Source: CAD feature listing. Evaluate the final solid. Frame: model axes, mm. A direction names the side the tool comes from. Round coordinates to 2 decimals unless told otherwise and drop trailing zeros. Order: outer loops, then holes, each group sorted by start corner. A loop starts at its lowest first (then second) coordinate and runs counter-clockwise, first axis right, second up. Notation, with made-up numbers: (-21.75, 57) -> (-17.75, 57) arc R33 cw to (-17.75, 94) -> close; hole circle Ø5 at (4.25, 23.25). An arc over 180 degrees is marked (long way). Write item = value, one per line. Start each with the question number.
(1) Contact query for flat-ended pins moving along their axis: pin 1 Ø1 at (x, z) = (9, 0) entering from +Y; pin 2 Ø0.5 at (x, z) = (15, 0) entering from -Y; pin 3 Ø1.5 at (y, z) = (6, 0) entering from +X. Output: stop coordinate, or through.
(2) Reachability of faces 1 (the face through (10.445, -2.742, -0.479)), 2 (the face through (1.42, -3.03, -0.48)), 3 (the face through (-2, 5, 0)) from +Z, -Z, +X, -X, +Y, -Y: full face, straight path, thin tool, end or side. Return the list, or none.
(3) Cut plane A-A on x = 6.5. Return the cut outline in (y, z).
(4) Cut plane B-B on z = 0.55. Return the cut outline in (x, y).
(5) Cut plane C-C on y = 3. Return the cut outline in (x, z), then the cut area to 3 significant figures.
(6) Ray query, line 1 (Y direction, x = 2.25, z = -1.05); line 2 (Y direction, x = 6.5, z = -1.1); line 3 (Y direction, x = 10, z = 0.15). Return the intervals inside material, ascending.
(7) Draft query along Y for faces 4 (the face through (2.545, 12.762, -0.479)), 5 (the face through (15, 5, 0)), 6 (the face through (13, 8, -2)), 7 (the face through (13, 3, -1)). Return one class per face: released by +Y, released by -Y, zero draft, split by the parting line, or undercut.
(8) Cut plane D-D on y = 12.5. Return the cut outline in (x, z), then the cut area to 3 significant figures.
from build123d import *

# Parameters (mm, degrees)
SKETCH009_R     = 9.5
PAD006_DEPTH    = 3
SKETCH010_R     = 6.8
POCKET003_DEPTH = 5
SKETCH013_W     = 1.6
SKETCH013_H     = 3
GROOVE_ANGLE    = -63
SKETCH014_W     = 1.6
SKETCH014_H     = 3
GROOVE001_ANGLE = -63


with BuildPart() as part:
    # Sketch009 → Pad006 (new body)
    with BuildSketch(Plane.XY.offset(1)):
        with Locations((6.5, 5)):
            Circle(SKETCH009_R)
    extrude(amount=-PAD006_DEPTH)

    # Sketch010 (on Face3 of Pad006) → Pocket003 (cut)
    with BuildSketch(Plane(origin=(0, 0, -2), x_dir=(1, 0, 0), z_dir=(0, 0, -1))):
        with Locations((6.5, -5)):
            Circle(SKETCH010_R)
    extrude(amount=-POCKET003_DEPTH, mode=Mode.SUBTRACT)

    # Sketch013 → Groove (revolve, cut)
    with BuildSketch(Plane(origin=(6.5, 5, 0), x_dir=(1, 0, 0), z_dir=(0, -1, 0))):
        with Locations((8.7, -0.5)):
            Rectangle(SKETCH013_W, SKETCH013_H)
    revolve(axis=Axis((6.5, 5, 0), (0, 0, 1)), revolution_arc=GROOVE_ANGLE, mode=Mode.SUBTRACT)

    # Sketch014 → Groove001 (revolve, cut)
    with BuildSketch(Plane(origin=(6.5, 5, 0), x_dir=(1, 0, 0), z_dir=(0, -1, 0))):
        with Locations((-8.7, -0.5)):
            Rectangle(SKETCH014_W, SKETCH014_H)
    revolve(axis=Axis((6.5, 5, 0), (0, 0, 1)), revolution_arc=GROOVE001_ANGLE, mode=Mode.SUBTRACT)


solid = part.part
Evaluation:
q1.pin_1 = 14.29
q1.pin_2 = 5
q1.pin_3 = 16
q2.face_1 = +Z, -Z, +X
q2.face_2 = +Z, -Z, -Y
q2.face_3 = +Z, -Z, -X, +Y
q3.outline = (-4.5, -2) -> (-1.8, -2) -> (-1.8, 1) -> (-4.5, 1) -> close; (11.8, -2) -> (14.5, -2) -> (14.5, 1) -> (11.8, 1) -> close
q4.outline = (-3, 5) arc R9.5 ccw to (10.81, -3.46) -> (10.09, -2.04) arc R7.9 ccw to (14.4, 5) -> (16, 5) arc R9.5 ccw to (2.19, 13.46) -> (2.91, 12.04) arc R7.9 ccw to (-1.4, 5) -> close; hole circle Ø13.6 at (6.5, 5)
q5.outline = (-2.79, -2) -> (0, -2) -> (0, 1) -> (-2.79, 1) -> close; (13, -2) -> (14.14, -2) -> (14.14, 1) -> (13, 1) -> close
q5.area = 11.8 mm^2
q6.line_1 = -3.5 to -0.31, 10.31 to 11.66, 13.34 to 13.5
q6.line_2 = -4.5 to -1.8, 11.8 to 14.5
q6.line_3 = -3.83 to -0.83, 10.83 to 13.83
q7.face_4 = undercut
q7.face_5 = released by -Y
q7.face_6 = zero draft
q7.face_7 = undercut
q8.outline = (2.68, -2) -> (12.33, -2) -> (12.33, 1) -> (2.68, 1) -> close
q8.area = 29.0 mm^2
